from build123d import *

# Parameters (mm, degrees)
SKETCH1_R           = 5.3
BOSS_EXTRUDE1_DEPTH = 1
SKETCH2_R           = 3.4
BOSS_EXTRUDE2_DEPTH = 6
SKETCH3_R           = 3
BOSS_EXTRUDE3_DEPTH = 14
SKETCH4_W           = 8
SKETCH4_H           = 1.2
CUT_EXTRUDE1_DEPTH  = 12
BOSS_EXTRUDE4_DEPTH = 0.6
BOSS_EXTRUDE5_DEPTH = 1
SKETCH7_R           = 8.25
BOSS_EXTRUDE6_DEPTH = 6
SKETCH8_W           = 3.5
SKETCH8_H           = 8
BOSS_EXTRUDE7_DEPTH = 0.5
SKETCH9_W           = 1
SKETCH9_H           = 2.5
BOSS_EXTRUDE8_DEPTH = 3


with BuildPart() as part:
    # Sketch1 → Boss-Extrude1 (new body)
    with BuildSketch(Plane(origin=(0, 0, 0), x_dir=(1, 0, 0), z_dir=(0, 1, 0))):
        with Locations(Location((0, 0, 0), (0, 0, 270))):
            Circle(SKETCH1_R)
    extrude(amount=-BOSS_EXTRUDE1_DEPTH)

    # Sketch2 → Boss-Extrude2 (add)
    with BuildSketch(Plane(origin=(0, 0, 0), x_dir=(1, 0, 0), z_dir=(0, 1, 0))):
        with Locations(Location((0, 0, 0), (0, 0, 270))):
            Circle(SKETCH2_R)
    extrude(amount=BOSS_EXTRUDE2_DEPTH)

    # Sketch3 → Boss-Extrude3 (add)
    with BuildSketch(Plane(origin=(0, 6, 0), x_dir=(1, 0, 0), z_dir=(0, 1, 0))):
        with Locations(Location((0, 0, 0), (0, 0, 270))):
            Circle(SKETCH3_R)
    extrude(amount=BOSS_EXTRUDE3_DEPTH)

    # Sketch4 → Cut-Extrude1 (cut)
    with BuildSketch(Plane(origin=(0, 20, 0), x_dir=(1, 0, 0), z_dir=(0, 1, 0))):
        Rectangle(SKETCH4_W, SKETCH4_H)
    extrude(amount=-CUT_EXTRUDE1_DEPTH, mode=Mode.SUBTRACT)

    # Sketch5 → Boss-Extrude4 (add)
    with BuildSketch(Plane.XZ.offset(1)):
        with BuildLine():
            Line((-6.480740698, 5.5), (6.480740698, 5.5))
            ThreePointArc((6.480740698, 5.5), (8.5, 0), (6.480740698, -5.5))
            Line((6.480740698, -5.5), (-6.480740698, -5.5))
            ThreePointArc((-6.480740698, -5.5), (-8.5, 0), (-6.480740698, 5.5))
        make_face()
    extrude(amount=BOSS_EXTRUDE4_DEPTH)

    # Sketch6 → Boss-Extrude5 (add)
    with BuildSketch(Plane.XZ.offset(1.6)):
        with BuildLine():
            Line((7.5, 4), (7.5, 11.5))
            Line((7.5, 11.5), (-7.5, 11.5))
            Line((-7.5, 11.5), (-7.5, 4))
            ThreePointArc((-7.5, 4), (0, -8.5), (7.5, 4))
        make_face()
    extrude(amount=BOSS_EXTRUDE5_DEPTH)

    # Sketch7 → Boss-Extrude6 (add)
    with BuildSketch(Plane.XZ.offset(2.6)):
        with Locations(Location((0, 0, 0), (0, 0, 270))):
            Circle(SKETCH7_R)
    extrude(amount=BOSS_EXTRUDE6_DEPTH)

    # Sketch8 → Boss-Extrude7 (add)
    with BuildSketch(Plane.XZ.offset(2.6)):
        with Locations((-5, 11.5)):
            Rectangle(SKETCH8_W, SKETCH8_H)
        with Locations((0, 11.5)):
            Rectangle(SKETCH8_W, SKETCH8_H)
        with Locations((5, 11.5)):
            Rectangle(SKETCH8_W, SKETCH8_H)
    extrude(amount=BOSS_EXTRUDE7_DEPTH)

    # Sketch9 → Boss-Extrude8 (add)
    with BuildSketch(Plane(origin=(0, -1, 0), x_dir=(1, 0, 0), z_dir=(0, 1, 0))):
        with Locations((-8, 0)):
            Rectangle(SKETCH9_W, SKETCH9_H)
    extrude(amount=BOSS_EXTRUDE8_DEPTH)


solid = part.part
The listing builds one solid part. Answer for the finished solid, in the listing's coordinates (mm). A direction names the side the tool comes from. Coordinates: 2 decimals unless noted, no trailing zeros. Loops run counter-clockwise (first coordinate to the right, second up) from the corner with the lowest first, then second, coordinate; pieces in that order, holes last.
1) Find the intervals of material crossed by L1, parallel to Z at x = 0, y = 12.75; L2, parallel to Y at x = 5, z = 1; L3, parallel to Y at x = 4, z = 5.25, in increasing order.
2) A tool of negligible diameter and unlimited length cuts with its end or side. For faces 4 (the face through (-5, -2.6, 14)), 5 (the face through (0, -1.6, -7)), 6 (the face through (-7.5, -2, 8)), 7 (the face through (-8, 0, 1.25)), 8 (the face through (-3, 6, 1)), from which of +Z, -Z, +X, -X, +Y, -Y can it reach the whole face along a straight path? Write none if from no direction.
3) Find section D-D on z = 9.75. Write down the section's boundary in (x, y).
4) Find section B-B on y = 14.5. Write down the section's boundary in (x, z).
5) Determine the mould class of faces 1 (the face through (0, 14, 0.6)), 2 (the face through (-8.5, 0, 0)), 3 (the face through (0, -2, 11.5)) for opening direction Z: pulls with the +Z half, pulls with the -Z half, needs draft (parallel to the pull), parting line crosses it, or undercut.
6) Flat-ended cylindrical pins translate along their axes: pin 1 Ø4 at (x, z) = (-6, -4.5) entering from +Y; pin 2 Ø1.1 at (x, z) = (-0.5, 13.5) entering from -Y; pin 3 Ø5 at (x, z) = (2.5, 11.5) entering from +Y. Find the tip coordinate at first contact, or state that the pin passes through.
7) Find section A-A on z = 13.5. Write down the section's boundary in (x, y).
Values:
1. L1: z = -3 to -0.6, 0.6 to 3
1. L2: y = -8.6 to 0
1. L3: y = -8.6 to -1
2. face 4: +Z, +X, -X, +Y
2. face 5: -Z, +X, -X, +Y
2. face 6: +Z, -X, +Y, -Y
2. face 7: +Z, -X, +Y
2. face 8: +Y
3. outline: (-7.5, -2.6) - (-6.75, -2.6) - (-6.75, -3.1) - (-3.25, -3.1) - (-3.25, -2.6) - (-1.75, -2.6) - (-1.75, -3.1) - (1.75, -3.1) - (1.75, -2.6) - (3.25, -2.6) - (3.25, -3.1) - (6.75, -3.1) - (6.75, -2.6) - (7.5, -2.6) - (7.5, -1.6) - (-7.5, -1.6) - close
4. outline: (-2.94, -0.6) arc R3 ccw to (2.94, -0.6) - close; (-2.94, 0.6) - (2.94, 0.6) arc R3 ccw to start
5. face 1: undercut
5. face 2: needs draft
5. face 3: pulls with the +Z half
6. pin 1: stops at y = -1
6. pin 2: stops at y = -3.1
6. pin 3: stops at y = -1.6
7. outline: (-6.75, -3.1) - (-3.25, -3.1) - (-3.25, -2.6) - (-6.75, -2.6) - close; (-1.75, -3.1) - (1.75, -3.1) - (1.75, -2.6) - (-1.75, -2.6) - close; (3.25, -3.1) - (6.75, -3.1) - (6.75, -2.6) - (3.25, -2.6) - close
